Geometry: see drawing. Coordinates: mm, zero at the bounding-box minimum. A direction names the side the tool comes from. Coordinates: 2 decimals unless noted, no trailing zeros. Loops run counter-clockwise (first coordinate to the right, second up) from the corner with the lowest first, then second, coordinate; pieces in that order, holes last. Notation, with made-up numbers: (44, -34.75) -> (59, -34.75) arc R34 cw to (59, 2.25) -> close; hole circle Ø11 at (-13.5, 7.5). An arc over 180 degrees is marked (long way). Put each result on its own line as item: value. Start each with the question number.
1) Material intervals for L1, parallel to X at y = 20, z = 4; L2, parallel to Z at x = 26.5, y = 54.5; L3, parallel to Z at x = 97, y = 43.5, sorted ascending.
2) Contact query for flat-ended pins moving along their axis: P1, Ø4, axis at x = 91, z = 18.5, coming from the +Y side; P2, Ø22, axis at x = 60.5, y = 61.5, coming from the -Z side. Output: stop coordinate, or through.
3) Cut plane C-C (y = 33). Return the cut outline in (x, z).
4) Cut plane D-D (y = 58). Return the cut outline in (x, z).
5) Set-up query: the marked faces 5, 6 and 7. Return all of +Z, -Z, +X, -X, +Y, -Y with unobstructed straight access to the full face (end or side cutting, diameter ignored); none if empty.
6) Pull-direction query (X, two-part tool) for the marked faces 1, 2, 3 and 4; classes: pulls with the +X half, pulls with the -X half, needs draft (parallel to the pull), parting line crosses it, or undercut.
7) Cut plane A-A (y = 15). Return the cut outline in (x, z), plus the area to 3 significant figures.
8) Cut plane B-B (z = 16). Return the cut outline in (x, y).
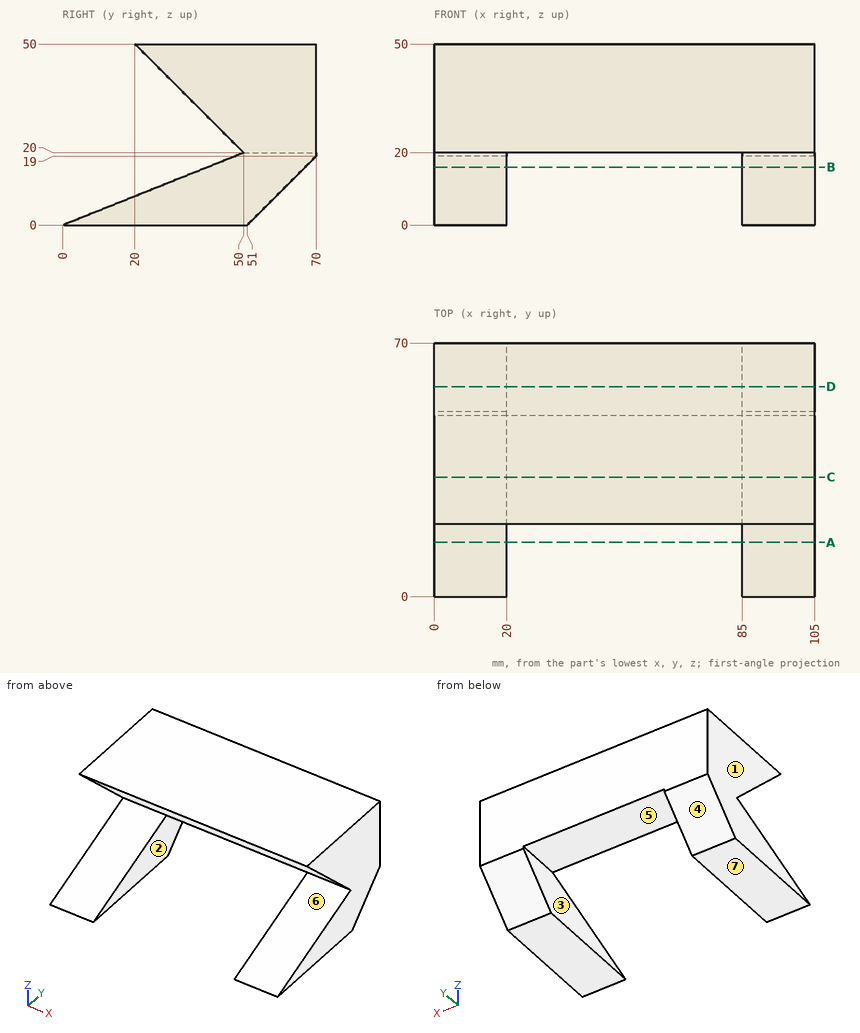
Results found:
1. L1: x = 0 to 20, 85 to 105
1. L2: z = 20 to 50
1. L3: z = 0 to 17.4, 26.5 to 50
2. P1: stops at y = 70
2. P2: stops at z = 20
3. outline: (0, 0) -> (20, 0) -> (20, 13.2) -> (0, 13.2) -> close; (0, 37) -> (105, 37) -> (105, 50) -> (0, 50) -> close; (85, 0) -> (105, 0) -> (105, 13.2) -> (85, 13.2) -> close
4. outline: (0, 7) -> (20, 7) -> (20, 20) -> (85, 20) -> (85, 7) -> (105, 7) -> (105, 50) -> (0, 50) -> close
5. face 5: -Z, +Y, -Y
5. face 6: +X, -X, -Y
5. face 7: -Z, +X, -X, +Y, -Y
6. face 1: pulls with the -X half
6. face 2: undercut
6. face 3: undercut
6. face 4: needs draft
7. outline: (0, 0) -> (20, 0) -> (20, 6) -> (0, 6) -> close; (85, 0) -> (105, 0) -> (105, 6) -> (85, 6) -> close
7. area: 240 mm2
8. outline: (0, 40) -> (20, 40) -> (20, 67) -> (0, 67) -> close; (85, 40) -> (105, 40) -> (105, 67) -> (85, 67) -> close
